Geometry: final body of the model. Coordinates: model frame, mm. A direction names the side the tool comes from. Give positions to 0.01 mm unless a question says otherwise; leave off trailing zeros. Loops run counter-clockwise (first coordinate to the right, second up) from the corner with the lowest first, then second, coordinate; pieces in that order, holes last. Notation, with made-up numbers: M -11.75,22.5 L 7.25,22.5 A22 cw 7.25,46.5 Z; hole C 34.5,57.5 d1. An arc over 180 degrees is marked long. Put each result on its own line as item: value.
```python
from build123d import *

# Parameters (mm, degrees)
CROQUIS1_W              = 50
CROQUIS1_H              = 10
CROQUIS1_R              = 2.1
SALIENTE_EXTRUIR1_DEPTH = 8
CROQUIS4_R              = 2.1
SALIENTE_EXTRUIR2_DEPTH = 25
CROQUIS5_R              = 15.800490208
CORTAR_EXTRUIR1_DEPTH   = 15
CORTAR_EXTRUIR2_DEPTH   = 2
CHAFL_N1_SIZE           = 3
CORTAR_EXTRUIR3_DEPTH   = 2
CHAFL_N2_SIZE           = 1
CHAFL_N2_SIZE_2         = 0.730640075


with BuildPart() as part:
    # Croquis1 → Saliente-Extruir1 (new body)
    with BuildSketch(Plane(origin=(0, 0, 0), x_dir=(1, 0, 0), z_dir=(0, 1, 0))):
        Rectangle(CROQUIS1_W, CROQUIS1_H)
        with Locations(Location((20, 0, 0), (0, 0, 270))):
            Circle(CROQUIS1_R, mode=Mode.SUBTRACT)
        with Locations(Location((-20, 0, 0), (0, 0, 90))):
            Circle(CROQUIS1_R, mode=Mode.SUBTRACT)
    extrude(amount=SALIENTE_EXTRUIR1_DEPTH)

    # Croquis4 → Saliente-Extruir2 (add, symmetric)
    with BuildSketch(Plane(origin=(0, 0, 0), x_dir=(0, 0, -1), z_dir=(1, 0, 0))):
        with BuildLine():
            Line((5, 8), (5, 0))
            Line((5, 0), (12.854829477, -15.59812982))
            ThreePointArc((12.854829477, -15.59812982), (25.037274777, -18.214970863), (24.999619637, -5.754697487))
            Line((24.999619637, -5.754697487), (10.01766425, 6.238969464))
            ThreePointArc((10.01766425, 6.238969464), (7.658861743, 7.54696071), (5, 8))
        make_face()
        with Locations((20, -12)):
            Circle(CROQUIS4_R, mode=Mode.SUBTRACT)
    extrude(amount=SALIENTE_EXTRUIR2_DEPTH, both=True)

    # Croquis5 → Cortar-Extruir1 (cut, symmetric)
    with BuildSketch(Plane(origin=(0, 0, 0), x_dir=(0, 0, -1), z_dir=(1, 0, 0))):
        with Locations((20, -12)):
            Circle(CROQUIS5_R)
    extrude(amount=CORTAR_EXTRUIR1_DEPTH, both=True, mode=Mode.SUBTRACT)

    # Croquis6 → Cortar-Extruir2 (cut, symmetric)
    with BuildSketch(Plane.ZY.offset(25)):
        Polygon((-16.016283143, -12), (-18.008141571, -8.55), (-21.991858429, -8.55), (-23.983716857, -12), (-21.991858429, -15.45), (-18.008141571, -15.45), align=None)
    cortar_extruir2 = extrude(amount=CORTAR_EXTRUIR2_DEPTH, both=True, mode=Mode.SUBTRACT)

    # Simetría1: Cortar-Extruir2 across plane
    add(cortar_extruir2.mirror(Plane(origin=(0, 0, 0), x_dir=(0, 0, 1), z_dir=(1, 0, 0))), mode=Mode.SUBTRACT)

    # Chaflán1
    chafl_n1_edges = [part.edges().sort_by_distance(p)[0] for p in [
        (25, 4, 5),
        (-25, 4, 5),
    ]]
    chamfer(chafl_n1_edges, length=CHAFL_N1_SIZE)

    # Croquis7 → Cortar-Extruir3 (cut, symmetric)
    with BuildSketch(Plane.XZ):
        Polygon((-16.016283143, 0), (-18.008141571, 3.45), (-21.991858429, 3.45), (-23.983716857, 0), (-21.991858429, -3.45), (-18.008141571, -3.45), align=None)
        Polygon((18.008141571, -3.45), (16.016283143, 0), (18.008141571, 3.45), (21.991858429, 3.45), (23.983716857, 0), (21.991858429, -3.45), align=None)
    extrude(amount=CORTAR_EXTRUIR3_DEPTH, both=True, mode=Mode.SUBTRACT)

    # Chaflán2
    # the kernel refuses this chamfer: 1, 0.730640075 mm, written as the material it takes off along each edge
    with BuildSketch(Plane(origin=(25, 8, -5), x_dir=(0, -1, 0), z_dir=(0, 0, 1))) as chafl_n2_piece_1:
        Polygon((CHAFL_N2_SIZE, 0), (0, -CHAFL_N2_SIZE), (0, 0), align=None)
    extrude(amount=9.571682988, mode=Mode.SUBTRACT)
    with BuildSketch(Plane(origin=(-25, 8, 4.571682988), x_dir=(1, 0, 0), z_dir=(0, 0, -1))) as chafl_n2_piece_2:
        Polygon((CHAFL_N2_SIZE, 0), (0, CHAFL_N2_SIZE), (0, 0), align=None)
    extrude(amount=9.571682988, mode=Mode.SUBTRACT)
    with BuildSketch(Plane(origin=(25, -12, -20), x_dir=(0, -0.44976622750296646, 0.8931463153357069), z_dir=(0, 0.8931463153357069, 0.44976622750296646))) as chafl_n2_piece_3:
        Polygon((8 - CHAFL_N2_SIZE, 0), (8, -CHAFL_N2_SIZE), (8, 0), align=None)
    revolve(axis=Axis((25, -12, -20), (1, 0, 0)), revolution_arc=204.592615825, mode=Mode.SUBTRACT)
    with BuildSketch(Plane(origin=(25, -5.754697487, -24.999619637), x_dir=(0, -0.7806628141857404, 0.6249524546296304), z_dir=(0, 0.6249524546296304, 0.7806628141857404)), Plane(origin=(-25, -5.754697487, -24.999619637), x_dir=(1, 0, 0), z_dir=(0, 0.6249524546296304, 0.7806628141857404))) as chafl_n2_piece_4:
        Polygon((CHAFL_N2_SIZE, 0), (0, -CHAFL_N2_SIZE), (0, 0), align=None)
    extrude(amount=19.191327055, mode=Mode.SUBTRACT)
    with BuildSketch(Plane(origin=(25, -0.028873577, -5), x_dir=(0, 0.7806628141857421, -0.6249524546296281), z_dir=(0, -0.6249524546296281, -0.7806628141857421))) as chafl_n2_piece_5:
        Polygon((8.028873577 - CHAFL_N2_SIZE, 0), (8.028873577, -CHAFL_N2_SIZE), (8.028873577, 0), align=None)
    revolve(axis=Axis((25, -0.028873577, -5), (1, 0, 0)), revolution_arc=38.678697835, mode=Mode.SUBTRACT)
    with BuildSketch(Plane(origin=(25, 2.296889185, -3.843343844), x_dir=(0, 0.44976622750296674, -0.8931463153357067), z_dir=(0, -0.8931463153357067, -0.44976622750296674))) as chafl_n2_piece_6_section:
        Polygon((CHAFL_N2_SIZE, 0), (0, -CHAFL_N2_SIZE), (0, 0), align=None)
    chafl_n2_piece_6 = extrude(amount=20.035932185, mode=Mode.PRIVATE)
    chafl_n2_piece_6 = split(chafl_n2_piece_6, bisect_by=Plane(origin=(25, 0, -3.843343844), z_dir=(0, -1, 0)), keep=Keep.TOP, mode=Mode.PRIVATE)
    add(chafl_n2_piece_6, mode=Mode.SUBTRACT)
    with BuildSketch(Plane(origin=(-25, -12, -20), x_dir=(0, -0.44976622750296646, 0.8931463153357069), z_dir=(0, 0.8931463153357069, 0.44976622750296646))) as chafl_n2_piece_7:
        Polygon((8 - CHAFL_N2_SIZE, 0), (8, CHAFL_N2_SIZE), (8, 0), align=None)
    revolve(axis=Axis((-25, -12, -20), (1, 0, 0)), revolution_arc=204.592615825, mode=Mode.SUBTRACT)
    with BuildSketch(Plane(origin=(-25, -0.028873577, -5), x_dir=(0, 0.7806628141857421, -0.6249524546296281), z_dir=(0, -0.6249524546296281, -0.7806628141857421))) as chafl_n2_piece_8:
        Polygon((8.028873577, CHAFL_N2_SIZE), (8.028873577 - CHAFL_N2_SIZE, 0), (8.028873577, 0), align=None)
    revolve(axis=Axis((-25, -0.028873577, -5), (1, 0, 0)), revolution_arc=38.678697835, mode=Mode.SUBTRACT)
    with BuildSketch(Plane(origin=(-25, 2.296889185, -3.843343844), x_dir=(1, 0, 0), z_dir=(0, -0.8931463153357067, -0.44976622750296674))) as chafl_n2_piece_9_section:
        Polygon((CHAFL_N2_SIZE, 0), (0, -CHAFL_N2_SIZE), (0, 0), align=None)
    chafl_n2_piece_9 = extrude(amount=20.035932185, mode=Mode.PRIVATE)
    chafl_n2_piece_9 = split(chafl_n2_piece_9, bisect_by=Plane(origin=(-25, 0, -3.843343844), z_dir=(0, -1, 0)), keep=Keep.TOP, mode=Mode.PRIVATE)
    add(chafl_n2_piece_9, mode=Mode.SUBTRACT)
    with BuildSketch(Plane(origin=(-15, -3.428524041, -6.72651927), x_dir=(0, 0.8931463153357074, 0.44976622750296513), z_dir=(1, 0, 0))) as chafl_n2_piece_10:
        with BuildLine():
            Line((CHAFL_N2_SIZE_2, 0), (0.494257976, -0.908692648))
            ThreePointArc((0.494257976, -0.908692648), (0.261545908, -0.46314506), (0, 0))
            Line((0, 0), (CHAFL_N2_SIZE_2, 0))
        make_face()
    extrude(amount=30, mode=Mode.SUBTRACT)
    with BuildSketch(Plane(origin=(-15, 2.760620634, -14.362662924), x_dir=(0, 0.6249524546296293, 0.7806628141857411), z_dir=(1, 0, 0))) as chafl_n2_piece_11:
        with BuildLine():
            Line((CHAFL_N2_SIZE_2, 0), (0.494257976, 0.908692648))
            ThreePointArc((0.494257976, 0.908692648), (0.261545908, 0.46314506), (0, 0))
            Line((0, 0), (CHAFL_N2_SIZE_2, 0))
        make_face()
    extrude(amount=30, mode=Mode.SUBTRACT)


solid = part.part
```
Item 1: Pin query (flat end, axial travel): pin 1 Ø5 at (x, z) = (-4, -16) entering from +Y; pin 2 Ø2 at (x, z) = (-24, -19.5) entering from -Y; pin 3 Ø1.5 at (x, z) = (-11.5, -1) entering from -Y; pin 4 Ø1.6 at (x, y) = (19.5, 1) entering from -Z. Return the tip coordinate at first contact, or that it passes through.
Output values:
pin 1: y = 3.45
pin 2: y = -20
pin 3: y = 0
pin 4: z = -17.56
Item 2: Mould query, pull axis X, two halves, no side actions, for faces 4 (the flat face through (-17, 1, -1.7)), 5 (the flat face through (24.5, 7.5, -1.1)), 6 (the flat face through (0, 8, 0)). Classes: pulls with the +X half, pulls with the -X half, needs draft (parallel to the pull), parting line crosses it, or undercut.
Output values:
face 4: undercut
face 5: pulls with the +X half
face 6: needs draft
Item 3: Set-up query: faces 1 (the flat face through (24, -10.3, -23)), 2 (the flat face through (-23, 1, -1.7)), 3 (the conical face through (-24.62, 6.95, -7.49)). Return all of +Z, -Z, +X, -X, +Y, -Y with unobstructed straight access to the full face (end or side cutting, diameter ignored); none if empty.
Output values:
face 1: +X
face 2: -Y
face 3: -Z, -X, +Y
Item 4: Section C-C on y = 4.5. Output: boundary loops of the cut face in (x, z), then the cut area to 3 significant figures.
Output values:
outline: M -25,-10.59 L -24,-12.19 L 24,-12.19 L 25,-10.59 L 25,2 L 22,5 L -22,5 L -25,2 Z; hole C -20,0 d4.2; hole C 20,0 d4.2
area: 821 mm²
Item 5: Section D-D on z = -20. Output: boundary loops of the cut face in (x, y).
Output values:
outline: M -25,-19 L -24,-20 L -15,-20 L -15,-14.1 L -23,-14.1 L -23,-15.45 L -25,-15.45 Z; M -25,-8.55 L -23,-8.55 L -23,-9.9 L -15,-9.9 L -15,-1.75 L -24,-1.75 L -25,-3.03 Z; M 15,-20 L 24,-20 L 25,-19 L 25,-15.45 L 23,-15.45 L 23,-14.1 L 15,-14.1 Z; M 15,-9.9 L 23,-9.9 L 23,-8.55 L 25,-8.55 L 25,-3.03 L 24,-1.75 L 15,-1.75 Z
Item 6: Section A-A on x = -20. Output: boundary loops of the cut face in (y, z), then the cut area to 3 significant figures.
Output values:
outline: M -15.6,-12.85 A8 ccw long -5.75,-25 L 6.24,-10.02 A8.03 ccw 8,-5 L 8,-2.1 L 2,-2.1 L 2,-3.45 L 0,-3.45 L 0,-5 Z; M 0,3.45 L 2,3.45 L 2,2.1 L 8,2.1 L 8,5 L 0,5 Z; hole C -12,-20 d4.2
area: 387 mm²
Item 7: Line query: probe 1 along X at (y, z) = (4.65, 0); probe 2 along X at (y, z) = (0, -11); probe 3 along Z at (x, y) = (-21, -12). Output: solid intervals per line, ascending. Write a range as [from, to].
Output values:
probe 1: [-25, -22.1], [-17.9, 17.9], [22.1, 25]
probe 2: [-25, -15], [15, 25]
probe 3: [-28, -22.1], [-17.9, -11.04]
Item 8: Section B-B on x = 11.5. Output: boundary loops of the cut face in (y, z).
Output values:
outline: M -2.78,-6.4 L -2.58,-7.32 A15.8 cw 2.36,-13.41 L 3.22,-13.79 L 6.24,-10.02 A8.03 ccw 8,-5 L 8,5 L 0,5 L 0,-5 Z
